Autodesk Inventor part; units mm, degrees
ref_plane "YZ Plane" through (0, 0, 0) normal (1, 0, 0) x (0, 1, 0)
ref_plane "XZ Plane" through (0, 0, 0) normal (0, 1, 0) x (-1, 0, 0)
ref_plane "XY Plane" through (0, 0, 0) normal (0, 0, 1) x (1, 0, 0)
sketch "草图1" plane through (0, 0, 0) normal (0, 0, 1) x (1, 0, 0)
  line L0 (-30, 425) -> (30, 425)
  line L1 (30, 425) -> (30, -425)
  line L2 (30, -425) -> (-30, -425)
  line L3 (-30, -425) -> (-30, 425)
  line L4 (-510, 0) -> (120, 0)
  line L5 (0, -595) -> (0, 595)
  line L6 (-420, 175) -> (-30, 175)
  line L7 (-30, 175) -> (-30, -125)
  line L8 (-30, -125) -> (-420, -125)
  line L9 (-420, -125) -> (-420, 175)
  point P0 (0, 0)
  point P1 (-30, 175)
  dimension "d0" = 60
  dimension "d1" = 850
  dimension "d2" = 390
  dimension "d3" = 250
  dimension "d4" = 300
extrude "拉伸1" add sketch "草图1" along normal mid plane 20
sketch "草图2" plane through (30, -425, 10) normal (1, 0, 0) x (0, 0, -1)
  line L0 (0, 0) -> (0, 850)
  line L1 (20, 850) -> (20, 0)
  line L2 (0, 500) -> (20, 500)
  line L3 (20, 500) -> (20, 400)
  line L4 (20, 400) -> (0, 400)
  line L5 (0, 400) -> (0, 500)
  line L6 (20, 850) -> (0, 850)
  point P0 (10, 425)
  point P1 (0, 400)
  dimension "d7" = 350
  dimension "d8" = 100
extrude "拉伸2" add sketch "草图2" along normal blind 25 contours L0 L2 L1 L4
sketch "草图3" plane through (-420, -125, 10) normal (-1, 0, 0) x (0, 0, 1)
  line L0 (-20, 0) -> (-20, 300)
  line L1 (0, 200) -> (0, 100)
  line L2 (-20, 200) -> (0, 200)
  line L3 (0, 200) -> (0, 100)
  line L4 (0, 100) -> (-20, 100)
  line L5 (-20, 100) -> (-20, 200)
  line L6 (-20, 550) -> (0, 550)
  point P0 (-10, 125)
  point P1 (-20, 100)
  point P2 (0, 200)
  dimension "d11" = 350
  dimension "d12" = 100
extrude "拉伸3" add sketch "草图3" along normal blind 25
properties part number "外壳挡板"
CAD build for the part. Positions are in the model's coordinates, mm. A direction names the side the tool comes from. Coordinates: 2 decimals unless noted, no trailing zeros. Write each loop counter-clockwise with the first axis right and the second up, starting at its lowest first coordinate (ties: lowest second). Pieces come first, ordered by that corner, then holes. Notation, with made-up numbers: M 14,-37.5 L 33,-37.5 A23 cw 33,-28.5 Z; hole C 76,-34 d4. An arc over 180 degrees is marked long. Answer as a JSON object with one key per item and string values. Group by question number.
1) Pin check, flat tips, straight feed: pin 1 Ø1.5 at (x, z) = (-62.5, -1.5) entering from +Y; pin 2 Ø8 at (y, z) = (-181.5, 4) entering from -X; pin 3 Ø10 at (x, z) = (-59.5, 0.5) entering from -Y. Stop position of each tip, or through.
2) Saw through at B-B (y = 131). Write the cut outline in (x, z).
3) Saw through at A-A (z = -7). Write the cut outline in (x, y).
4) Tool access for faces 1 (the face through (30, 252, 0)), 2 (the face through (-228, 175, 0)), 3 (the face through (42, -25, 0)), 4 (the face through (-420, -76, 0)): list every direction of +Z, -Z, +X, -X, +Y, -Y with a clear straight run to the whole face (end or side of a thin tool).
5) Wall check: line 1 (X direction, y = -205, z = -8.5); line 2 (Y direction, x = -292, z = 8.25); line 3 (X direction, y = 146, z = 7.75). Give the ranges that are in metal, low to high. Write a range as from..to.
6) Saw through at C-C (x = -317). Write the cut outline in (y, z).
Values follow:
{
 "1": {"pin 1": "stops at y = 175", "pin 2": "stops at x = -30", "pin 3": "stops at y = -125"},
 "2": {"outline": "M -420,-10 L 30,-10 L 30,10 L -420,10 Z"},
 "3": {"outline": "M -445,-25 L -420,-25 L -420,-125 L -30,-125 L -30,-425 L 30,-425 L 30,-25 L 55,-25 L 55,75 L 30,75 L 30,425 L -30,425 L -30,175 L -420,175 L -420,75 L -445,75 Z"},
 "4": {"face 1": "+Z, -Z, +X, +Y", "face 2": "+Z, -Z, -X, +Y", "face 3": "+Z, -Z, +X, -Y", "face 4": "+Z, -Z, -X, -Y"},
 "5": {"line 1": "x = -30..30", "line 2": "y = -125..175", "line 3": "x = -420..30"},
 "6": {"outline": "M -125,-10 L 175,-10 L 175,10 L -125,10 Z"}
}
